The model under review builds one solid part; all positions refer to its coordinate system, in mm. A direction names the side the tool comes from. Coordinates: 2 decimals unless noted, no trailing zeros. Loops run counter-clockwise (first coordinate to the right, second up) from the corner with the lowest first, then second, coordinate; pieces in that order, holes last. Notation, with made-up numbers: (85.25, 19.5) -> (142.25, 19.5) arc R33 ccw to (142.25, 54.5) -> close; hole circle Ø8 at (8.25, 29.25). An arc over 180 degrees is marked (long way). One line per question, with ' | ' between items. Start each with the question number.
Autodesk Inventor part; units mm, degrees
ref_plane "YZ Plane" through (0, 0, 0) normal (1, 0, 0) x (0, 1, 0)
ref_plane "XZ Plane" through (0, 0, 0) normal (0, 1, 0) x (-1, 0, 0)
ref_plane "XY Plane" through (0, 0, 0) normal (0, 0, 1) x (1, 0, 0)
sketch "Esquisse1" plane through (0, 0, 0) normal (0, 0, 1) x (1, 0, 0)
  line L0 (0, 0) -> (23.4, 0)
  line L1 (23.4, 0) -> (23.4, 6.2)
  line L2 (11.4, 18.2) -> (0, 18.2)
  line L3 (0, 18.2) -> (0, 0)
  arc A0 (23.4, 6.2) -> (11.4, 18.2) centre (11.4, 6.2) ccw
  dimension "d0" = 18.2
  dimension "d1" = 23.4
  dimension "d2" = 12
extrude "Extrusion1" add sketch "Esquisse1" along normal blind 2
sketch "Esquisse2" plane through (0, 0, 0) normal (0, -1, 0) x (1, 0, 0)
  line L0 (0, 2) -> (23.4, 2)
  line L1 (0, 2) -> (23.4, 2)
  line L2 (23.4, 2) -> (23.4, 11)
  line L3 (23.4, 11) -> (0, 11)
  line L4 (0, 11) -> (0, 2)
  point P0 (0, 0)
  dimension "d5" = 9
extrude "Extrusion2" add sketch "Esquisse2" against normal blind 2
sketch "Esquisse3" plane through (0, 0, 11) normal (0, 0, 1) x (1, 0, 0)
  line L0 (0, 2) -> (23.4, 2)
  line L1 (23.4, 2) -> (0, 2)
  line L2 (0, 2) -> (0, 18.2)
  line L3 (0, 18.2) -> (11.4, 18.2)
  line L4 (23.4, 6.2) -> (23.4, 2)
  arc A0 (23.4, 6.2) -> (11.4, 18.2) centre (11.4, 6.2) ccw
  point P0 (0, 0)
  dimension "d8" = 16.2
  dimension "d9" = 12
extrude "Extrusion3" add sketch "Esquisse3" against normal blind 2
sketch "Esquisse4" plane through (0, 0, 11) normal (0, 0, 1) x (1, 0, 0)
  circle A0 centre (3.39, 9.1) radius 2
  line L0 (23.4, 0) -> (0, 0)
  line L1 (23.4, 0) -> (23.4, 6.2)
  line L2 (0, 0) -> (0, 18.2)
  dimension "d12" = 9.1
  dimension "d14" = 4
  dimension "d19" = 3.39
extrude "Extrusion4" cut sketch "Esquisse4" against normal blind 2
sketch "Esquisse5" plane through (0, 0, 0) normal (0, 0, -1) x (-1, 0, 0)
  circle A0 centre (-3.39, 9.1) radius 2
  circle A1 centre (-3.39, 9.1) radius 2
  point P0 (0, 0)
extrude "Extrusion5" cut sketch "Esquisse5" against normal blind 2
properties part number "Finger2" material "Plastique ABS"
1) Wall thickness on L1, parallel to Z at x = 13.25, y = 7.5; L2, parallel to Y at x = 3.39, z = 10.45; L3, parallel to Y at x = 7.5, z = 8.25: over which ranges is each line inside the solid? List them lowest first.
2) Mouldability with a two-part tool opening along Y and no side actions: class faces 3 (the face through (6, 18.2, 1)), 4 (the face through (1.482, 9.701, 0.986)), 5 (the face through (23.4, 1.8, 5.6)) as +Y half, -Y half, draft (parallel to the pull), parting line (faces both ways), or undercut.
3) Machinability: for faces 1 (the face through (12, 9, 11)), 2 (the face through (12, 2, 6)), which of the approach directions +Z, -Z, +X, -X, +Y, -Y give a long, thin tool a straight path to every point of the face, cutting with its end or side? Answer none if there is none.
4) Consider section C-C, the plane z = 1.5. Write out the cut boundary in (x, y).
5) Consider section A-A, the plane x = 3.39. Write out the cut boundary in (y, z), plus the area to 3 significant figures.
6) Consider section B-B, the plane y = 10.25. Write out the cut boundary in (x, z), plus the area to 3 significant figures.
7) Consider section D-D, the plane x = 7.5. Write out the cut boundary in (y, z), plus the area to 3 significant figures.
Filled sheet:
1) L1: 0 to 2, 9 to 11 | L2: 0 to 7.1, 11.1 to 18.2 | L3: 0 to 2
2) face 3: +Y half | face 4: undercut | face 5: draft
3) face 1: +Z, +X, -X, +Y, -Y | face 2: +X, -X, +Y
4) outline: (0, 0) -> (23.4, 0) -> (23.4, 6.2) arc R12 ccw to (11.4, 18.2) -> (0, 18.2) -> close; hole circle Ø4 at (3.39, 9.1)
5) outline: (0, 0) -> (7.1, 0) -> (7.1, 2) -> (2, 2) -> (2, 9) -> (7.1, 9) -> (7.1, 11) -> (0, 11) -> close; (11.1, 0) -> (18.2, 0) -> (18.2, 2) -> (11.1, 2) -> close; (11.1, 9) -> (18.2, 9) -> (18.2, 11) -> (11.1, 11) -> close | area: 70.8 mm^2
6) outline: (0, 0) -> (1.75, 0) -> (1.75, 2) -> (0, 2) -> close; (0, 9) -> (1.75, 9) -> (1.75, 11) -> (0, 11) -> close; (5.03, 0) -> (22.7, 0) -> (22.7, 2) -> (5.03, 2) -> close; (5.03, 9) -> (22.7, 9) -> (22.7, 11) -> (5.03, 11) -> close | area: 77.7 mm^2
7) outline: (0, 0) -> (18.2, 0) -> (18.2, 2) -> (2, 2) -> (2, 9) -> (18.2, 9) -> (18.2, 11) -> (0, 11) -> close | area: 86.8 mm^2
